Here's how the part is built. I have some questions about the finished solid (model axes, mm). Face numbers are marked on the shaded views. A direction names the side the tool comes from. Round coordinates to 2 decimals unless told otherwise and drop trailing zeros. Loops run counter-clockwise (first coordinate to the right, second up) from the corner with the lowest first, then second, coordinate; pieces in that order, holes last. Notation, with made-up numbers: M 3.25,40 L 21.25,40 A37 ccw 21.25,78 Z; hole C 83.25,-33 d5. An arc over 180 degrees is marked long. Answer as CSV lines item,"result".
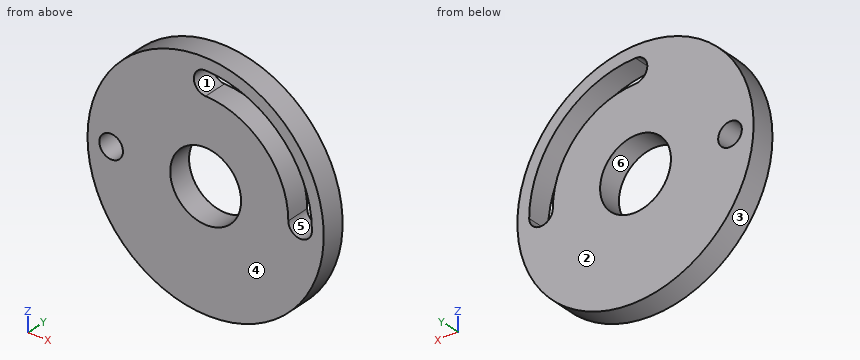
Autodesk Inventor part; units mm, degrees
ref_plane "YZ Plane" through (0, 0, 0) normal (1, 0, 0) x (0, 1, 0)
ref_plane "XZ Plane" through (0, 0, 0) normal (0, 1, 0) x (-1, 0, 0)
ref_plane "XY Plane" through (0, 0, 0) normal (0, 0, 1) x (1, 0, 0)
sketch "Sketch1" plane through (0, 0, 0) normal (0, 1, 0) x (-1, 0, 0)
  circle A0 centre (0, 0) radius 25
  dimension "d0" = 50
extrude "Extrusion1" add sketch "Sketch1" along normal blind 5
sketch "Sketch2" plane through (0, 5, 0) normal (0, 1, 0) x (1, 0, 0)
  circle A0 centre (0, 0) radius 7.5
  dimension "d3" = 15
extrude "Extrusion2" cut sketch "Sketch2" against normal through all
sketch "Sketch4" plane through (0, 0, 0) normal (0, -1, 0) x (1, 0, 0)
  circle A0 centre (0, 0) radius 20 construction
  arc A1 (0, 22.5) -> (0, 17.5) centre (0, 20) ccw
  arc A2 (17.5, 0) -> (22.5, 0) centre (20, 0) ccw
  arc A3 (22.5, 0) -> (0, 22.5) centre (0, 0) ccw
  arc A4 (17.5, 0) -> (0, 17.5) centre (0, 0) ccw
  circle A5 centre (0, 0) radius 7.5
  circle A6 centre (0, 0) radius 25
  dimension "d9" = 5
  dimension "d10" = 5
  dimension "d11" = 90
extrude "Extrusion3" cut sketch "Sketch4" against normal through all contours A3 A2 A4 A1
sketch "Sketch8" plane through (0, 0, 0) normal (0, -1, 0) x (1, 0, 0)
  circle A0 centre (0, 0) radius 20 construction
  arc A1 (22.5, 0) -> (0, 22.5) centre (0, 0) ccw
  arc A2 (17.5, 0) -> (22.5, 0) centre (20, 0) ccw
  arc A3 (17.5, 0) -> (0, 17.5) centre (0, 0) ccw
  arc A4 (0, 22.5) -> (0, 17.5) centre (0, 20) ccw
  circle A5 centre (0, 0) radius 7.5
  circle A6 centre (0, 0) radius 25
  arc A7 (17.5, 0) -> (0, 17.5) centre (0, 0) ccw
  circle A8 centre (0, 0) radius 25
  circle A9 centre (-20, 0) radius 2.5
  dimension "d15" = 5
extrude "Extrusion4" cut sketch "Sketch8" against normal through all contours A9
equation "\"kat_promienia\" = 30deg"
properties part number "sprzeglo_02"
1. I want a section at B-B, the plane z = 20. Please give me the cut outline in (x, y), and give its area (3 significant figures).
Evaluation:
outline,"M -15,0 L -2.5,0 L -2.5,5 L -15,5 Z; M 10.31,0 L 15,0 L 15,5 L 10.31,5 Z"
area,"86.0 mm²"
2. For P1, Ø2, axis at x = 18, z = 2, coming from the +Y side; P2, Ø12, axis at x = 0, z = 0, coming from the -Y side, each with a flat end and sliding along its axis, tell me the tip position at first contact or that it passes through.
Evaluation:
P1,"stops at y = 5"
P2,"passes through"
3. If I drill on line 1 (Z direction, x = 0, y = 1.2); line 2 (X direction, y = 1.4, z = 4); line 3 (X direction, y = 3.1, z = 4.5), over which ranges is the centre line in solid material (lowest first)? Write a range as [from, to].
Evaluation:
line 1,"z = [-25, -7.5], [7.5, 17.5], [22.5, 25]"
line 2,"x = [-24.68, -6.34], [6.34, 17.04], [22.14, 24.68]"
line 3,"x = [-24.59, -6], [6, 16.91], [22.05, 24.59]"
4. Which directions (+Z, -Z, +X, -X, +Y, -Y) give clear straight access to the entire face, cutting with the end or side of a thin tool? Please do the marked faces 1 and 2.
Evaluation:
face 1,"+Y, -Y"
face 2,"+Z, -Z, +X, -X, +Y"
5. I want a section at A-A, the plane x = -20. Please give me the cut outline in (y, z).
Evaluation:
outline,"M 0,-15 L 5,-15 L 5,-2.5 L 0,-2.5 Z; M 0,2.5 L 5,2.5 L 5,15 L 0,15 Z"
6. I want a section at C-C, the plane y = 4.4. Please give me the cut outline in (x, z), and give its area (3 significant figures).
Evaluation:
outline,"C 0,0 d50; hole C -20,0 d5; hole C 0,0 d15; hole M 0,17.5 A17.5 cw 17.5,0 A2.5 ccw 22.5,0 A22.5 ccw 0,22.5 A2.5 ccw Z"
area,"1,590 mm²"
7. We'd pull the mould along X, two halves only. Please class the marked faces 3, 4, 5 and 6: pulls with the +X half, pulls with the -X half, needs draft (parallel to the pull), parting line crosses it, or undercut.
Evaluation:
face 3,"parting line crosses it"
face 4,"needs draft"
face 5,"undercut"
face 6,"undercut"
8. I want a section at D-D, the plane x = 1.5. Please give me the cut outline in (y, z), and give its area (3 significant figures).
Evaluation:
outline,"M 0,-24.95 L 5,-24.95 L 5,-7.35 L 0,-7.35 Z; M 0,7.35 L 5,7.35 L 5,17.44 L 0,17.44 Z; M 0,22.45 L 5,22.45 L 5,24.95 L 0,24.95 Z"
area,"151 mm²"
